from build123d import *

# Parameters (mm, degrees)
SKETCH1_R           = 47.5
SKETCH1_R_2         = 39
BOSS_EXTRUDE1_DEPTH = 15
BOSS_EXTRUDE2_START = 8
SKETCH4_R           = 47.5
SKETCH4_R_2         = 20
BOSS_EXTRUDE2_DEPTH = 8
SKETCH5_R           = 23.5
CUT_EXTRUDE3_DEPTH  = 7
SKETCH6_R           = 1.9
CUT_EXTRUDE4_DEPTH  = 72.003521039
CUT_EXTRUDE5_DEPTH  = 5


with BuildPart() as part:
    # Sketch1 → Boss-Extrude1 (new body)
    with BuildSketch(Plane.XY):
        Circle(SKETCH1_R)
        Circle(SKETCH1_R_2, mode=Mode.SUBTRACT)
    extrude(amount=BOSS_EXTRUDE1_DEPTH)

    # Sketch4 → Boss-Extrude2 (add)
    with BuildSketch(Plane(origin=(0, 0, 0), x_dir=(-1, 0, 0), z_dir=(0, 0, -1)).offset(BOSS_EXTRUDE2_START)):
        Circle(SKETCH4_R)
        Circle(SKETCH4_R_2, mode=Mode.SUBTRACT)
    extrude(amount=-BOSS_EXTRUDE2_DEPTH)

    # Sketch5 → Cut-Extrude3 (cut)
    with BuildSketch(Plane.XY):
        Circle(SKETCH5_R)
    extrude(amount=-CUT_EXTRUDE3_DEPTH, mode=Mode.SUBTRACT)

    # Sketch6 → Cut-Extrude4 (cut, through all)
    with BuildSketch(Plane.XY.offset(15)):
        with Locations((44, 0)):
            Circle(SKETCH6_R)
        with Locations((22, -38.105117767)):
            Circle(SKETCH6_R)
        with Locations((-22, -38.105117767)):
            Circle(SKETCH6_R)
        with Locations((-44, 0)):
            Circle(SKETCH6_R)
        with Locations((-22, 38.105117767)):
            Circle(SKETCH6_R)
        with Locations((22, 38.105117767)):
            Circle(SKETCH6_R)
    extrude(amount=-CUT_EXTRUDE4_DEPTH, mode=Mode.SUBTRACT)

    # Sketch7 → Cut-Extrude5 (cut)
    with BuildSketch(Plane(origin=(0, 0, -8), x_dir=(-1, 0, 0), z_dir=(0, 0, -1))):
        with BuildLine():
            Line((44, 3.5), (47.370877129, 3.5))
            ThreePointArc((47.370877129, 3.5), (47.5, 0), (47.370877129, -3.5))
            Line((47.370877129, -3.5), (44, -3.5))
            ThreePointArc((44, -3.5), (40.5, 0), (44, 3.5))
        make_face()
        with BuildLine():
            Line((25.031088913, -36.355117767), (26.716527478, -39.274382994))
            ThreePointArc((26.716527478, -39.274382994), (23.75, -41.13620668), (20.654349651, -42.774382994))
            Line((20.654349651, -42.774382994), (18.968911087, -39.855117767))
            ThreePointArc((18.968911087, -39.855117767), (20.25, -35.074028853), (25.031088913, -36.355117767))
        make_face()
        with BuildLine():
            Line((-18.968911087, -39.855117767), (-20.654349651, -42.774382994))
            ThreePointArc((-20.654349651, -42.774382994), (-23.75, -41.13620668), (-26.716527478, -39.274382994))
            Line((-26.716527478, -39.274382994), (-25.031088913, -36.355117767))
            ThreePointArc((-25.031088913, -36.355117767), (-20.25, -35.074028853), (-18.968911087, -39.855117767))
        make_face()
        with BuildLine():
            Line((-44, -3.5), (-47.370877129, -3.5))
            ThreePointArc((-47.370877129, -3.5), (-47.5, 0), (-47.370877129, 3.5))
            Line((-47.370877129, 3.5), (-44, 3.5))
            ThreePointArc((-44, 3.5), (-40.5, 0), (-44, -3.5))
        make_face()
        with BuildLine():
            Line((-25.031088913, 36.355117767), (-26.716527478, 39.274382994))
            ThreePointArc((-26.716527478, 39.274382994), (-23.75, 41.13620668), (-20.654349651, 42.774382994))
            Line((-20.654349651, 42.774382994), (-18.968911087, 39.855117767))
            ThreePointArc((-18.968911087, 39.855117767), (-20.25, 35.074028853), (-25.031088913, 36.355117767))
        make_face()
        with BuildLine():
            Line((18.968911087, 39.855117767), (20.654349651, 42.774382994))
            ThreePointArc((20.654349651, 42.774382994), (23.75, 41.13620668), (26.716527478, 39.274382994))
            Line((26.716527478, 39.274382994), (25.031088913, 36.355117767))
            ThreePointArc((25.031088913, 36.355117767), (20.25, 35.074028853), (18.968911087, 39.855117767))
        make_face()
    extrude(amount=-CUT_EXTRUDE5_DEPTH, mode=Mode.SUBTRACT)


solid = part.part
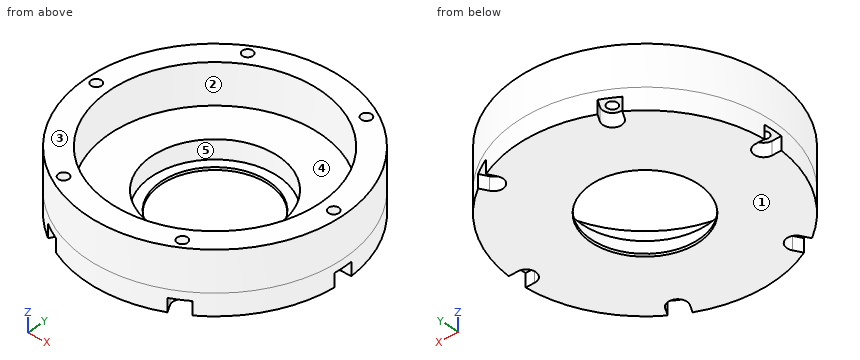
Could you check a few things on this model? Use its own coordinates, in mm. Face numbers are marked on the shaded views. A direction names the side the tool comes from. Coordinates: 2 decimals unless noted, no trailing zeros. Order: outer loops, then holes, each group sorted by start corner. A loop starts at its lowest first (then second) coordinate and runs counter-clockwise, first axis right, second up. Notation, with made-up numbers: (84, -31.5) -> (135, -31.5) arc R14 ccw to (135, -6.5) -> close; hole circle Ø5 at (23, 77.25). An arc over 180 degrees is marked (long way). One line per item, written item: value. Start each with the question number.
1) Which directions (+Z, -Z, +X, -X, +Y, -Y) give clear straight access to the entire face, cutting with the end or side of a thin tool? Please do the marked faces 1 and 2.
2) Imagine slicing it at C-C on x = 22. List the corners of the cut face in (y, z) for me.
3) Imagine slicing it at B-B on x = 0. List the corners of the cut face in (y, z) for me.
4) Imagine slicing it at A-A on y = 0. List the corners of the cut face in (x, z) for me, plus the area to 3 significant figures.
5) I'm going to push flat-ended pins straight in: pin 1 (6.5 mm diameter, centred on x = 20.5, y = 39, fed in from -Z); pin 2 (2 mm diameter, centred on y = 12.5, z = -2.5, fed in from +X); pin 3 (6 mm diameter, centred on x = 34.5, y = 10, fed in from +Z); pin 4 (8 mm diameter, centred on x = -6.5, z = -1.5, fed in from -Y). Where does each tip first touch, or does it pass through?
6) If I drill on L1, parallel to Y at x = 22, z = 3; L2, parallel to X at y = 7, z = 6.25; L3, parallel to Z at x = 37, y = 6, over which ranges is the centre line in solid material (lowest first)? Write a range as [from, to].
7) We'd pull the mould along X, two halves only. Please class the marked faces 3, 4 and 5: +X half, -X half, draft (parallel to the pull), parting line (faces both ways), or undercut.
8) Imagine slicing it at D-D on y = 12.5. List the corners of the cut face in (x, z) for me.
Answer list:
1. face 1: -Z, +X, -X, +Y, -Y
1. face 2: +Z
2. outline: (-42.1, -3) -> (-40.01, -3) -> (-40.01, 15) -> (-42.1, 15) -> close; (-36.21, -3) -> (-34.61, -3) -> (-34.61, -8) -> (34.61, -8) -> (34.61, -3) -> (36.21, -3) -> (36.21, 15) -> (32.2, 15) -> (32.2, 0) -> (8.26, 0) -> (8.26, -7) -> (-8.26, -7) -> (-8.26, 0) -> (-32.2, 0) -> (-32.2, 15) -> (-36.21, 15) -> close; (40.01, -3) -> (42.1, -3) -> (42.1, 15) -> (40.01, 15) -> close
3. outline: (-47.5, -8) -> (-20, -8) -> (-20, -7) -> (-23.5, -7) -> (-23.5, 0) -> (-39, 0) -> (-39, 15) -> (-47.5, 15) -> close; (20, -8) -> (47.5, -8) -> (47.5, 15) -> (39, 15) -> (39, 0) -> (23.5, 0) -> (23.5, -7) -> (20, -7) -> close
4. outline: (-47.5, -3) -> (-45.9, -3) -> (-45.9, 15) -> (-47.5, 15) -> close; (-42.1, -3) -> (-40.5, -3) -> (-40.5, -8) -> (-20, -8) -> (-20, -7) -> (-23.5, -7) -> (-23.5, 0) -> (-39, 0) -> (-39, 15) -> (-42.1, 15) -> close; (20, -8) -> (40.5, -8) -> (40.5, -3) -> (42.1, -3) -> (42.1, 15) -> (39, 15) -> (39, 0) -> (23.5, 0) -> (23.5, -7) -> (20, -7) -> close; (45.9, -3) -> (47.5, -3) -> (47.5, 15) -> (45.9, 15) -> close
4. area: 439 mm2
5. pin 1: stops at z = -8
5. pin 2: stops at x = 46.09
5. pin 3: stops at z = 0
5. pin 4: stops at y = -47.43
6. L1: y = [-42.1, -40.01], [-36.21, -32.2], [32.2, 36.21], [40.01, 42.1]
6. L2: x = [-46.98, -38.37], [38.37, 46.98]
6. L3: z = [-8, 0]
7. face 3: draft
7. face 4: undercut
7. face 5: undercut
8. outline: (-45.83, -8) -> (-15.61, -8) -> (-15.61, -7) -> (-19.9, -7) -> (-19.9, 0) -> (-36.94, 0) -> (-36.94, 15) -> (-45.83, 15) -> close; (15.61, -8) -> (45.83, -8) -> (45.83, 15) -> (36.94, 15) -> (36.94, 0) -> (19.9, 0) -> (19.9, -7) -> (15.61, -7) -> close
